Geometry check sheet. Reference: the model listing, model coordinates, mm. A direction names the side the tool comes from. Coordinates: 2 decimals unless noted, no trailing zeros. Write each loop counter-clockwise with the first axis right and the second up, starting at its lowest first coordinate (ties: lowest second). Pieces come first, ordered by that corner, then holes. Notation, with made-up numbers: M 44,59.5 L 83,59.5 A8 cw 83,63.5 Z; hole C 71,-5 d10. An arc over 180 degrees is marked long. Write each question's results on one line, items separated by ' | '.
```python
from build123d import *

# Parameters (mm, degrees)
SKETCH1_W           = 66
SKETCH1_H           = 54
BOSS_EXTRUDE1_DEPTH = 5
SKETCH2_R           = 2.5
SKETCH2_R_2         = 0.75
BOSS_EXTRUDE2_DEPTH = 4
SKETCH2_2_R         = 0.75
CUT_EXTRUDE1_DEPTH  = 4
CUT_EXTRUDE2_DEPTH  = 14
SKETCH4_R           = 1.6
SKETCH4_R_2         = 0.75
CUT_EXTRUDE3_DEPTH  = 5
CHAMFER1_SIZE       = 2
CUT_EXTRUDE4_START  = -66
SKETCH5_R           = 1.6
CUT_EXTRUDE4_DEPTH  = 10
SKETCH6_W           = 9.6
SKETCH6_H           = 16.5
CUT_EXTRUDE5_DEPTH  = 2.54


with BuildPart() as part:
    # Sketch1 → Boss-Extrude1 (new body)
    with BuildSketch(Plane.XY):
        Rectangle(SKETCH1_W, SKETCH1_H)
    extrude(amount=BOSS_EXTRUDE1_DEPTH)

    # Sketch2 → Boss-Extrude2 (add)
    with BuildSketch(Plane.XY.offset(5)):
        with Locations((28, -23)):
            Circle(SKETCH2_R)
        with Locations((28, -23)):
            Circle(SKETCH2_R_2, mode=Mode.SUBTRACT)
        with Locations((-28, -23)):
            Circle(SKETCH2_R)
        with Locations((-28, -23)):
            Circle(SKETCH2_R_2, mode=Mode.SUBTRACT)
        with Locations((-28, 23)):
            Circle(SKETCH2_R)
        with Locations((-28, 23)):
            Circle(SKETCH2_R_2, mode=Mode.SUBTRACT)
        with Locations((28, 23)):
            Circle(SKETCH2_R)
        with Locations((28, 23)):
            Circle(SKETCH2_R_2, mode=Mode.SUBTRACT)
        with BuildLine():
            Line((-25.5, 4), (-25.5, -4))
            ThreePointArc((-25.5, -4), (-28, -6.5), (-30.5, -4))
            Line((-30.5, -4), (-30.5, 4))
            ThreePointArc((-30.5, 4), (-28, 6.5), (-25.5, 4))
        make_face()
        with Locations((-28, -4)):
            Circle(SKETCH2_R_2, mode=Mode.SUBTRACT)
        with Locations((-28, 4)):
            Circle(SKETCH2_R_2, mode=Mode.SUBTRACT)
        with BuildLine():
            Line((25.5, 4), (25.5, -4))
            ThreePointArc((25.5, -4), (28, -6.5), (30.5, -4))
            Line((30.5, -4), (30.5, 4))
            ThreePointArc((30.5, 4), (28, 6.5), (25.5, 4))
        make_face()
        with Locations((28, -4)):
            Circle(SKETCH2_R_2, mode=Mode.SUBTRACT)
        with Locations((28, 4)):
            Circle(SKETCH2_R_2, mode=Mode.SUBTRACT)
    extrude(amount=BOSS_EXTRUDE2_DEPTH)

    # Sketch2<2> → Cut-Extrude1 (cut)
    with BuildSketch(Plane.XY.offset(5)):
        with Locations((-28, 23)):
            Circle(SKETCH2_2_R)
        with Locations((28, 23)):
            Circle(SKETCH2_2_R)
        with Locations((28, 4)):
            Circle(SKETCH2_2_R)
        with Locations((28, -4)):
            Circle(SKETCH2_2_R)
        with Locations((28, -23)):
            Circle(SKETCH2_2_R)
        with Locations((-28, -23)):
            Circle(SKETCH2_2_R)
        with Locations((-28, 4)):
            Circle(SKETCH2_2_R)
        with Locations((-28, -4)):
            Circle(SKETCH2_2_R)
    extrude(amount=-CUT_EXTRUDE1_DEPTH, mode=Mode.SUBTRACT)

    # Sketch3 → Cut-Extrude2 (cut)
    with BuildSketch(Plane.XY.offset(5)):
        with BuildLine():
            Line((-16.040925592, 12.723978191), (-5.394585654, 1.367882258))
            ThreePointArc((-5.394585654, 1.367882258), (-4.853660062, 0), (-5.394585654, -1.367882258))
            Line((-5.394585654, -1.367882258), (-16.040925592, -12.723978191))
            ThreePointArc((-16.040925592, -12.723978191), (-18.235476439, -13.21595464), (-19.5, -11.356095934))
            Line((-19.5, -11.356095934), (-19.5, 11.356095934))
            ThreePointArc((-19.5, 11.356095934), (-18.235476439, 13.21595464), (-16.040925592, 12.723978191))
        make_face()
        with BuildLine():
            Line((-10.958839938, 21), (10.958839938, 21))
            ThreePointArc((10.958839938, 21), (12.794019018, 19.795058326), (12.417914346, 17.632117742))
            Line((12.417914346, 17.632117742), (1.459074408, 5.942688475))
            ThreePointArc((1.459074408, 5.942688475), (0, 5.310570733), (-1.459074408, 5.942688475))
            Line((-1.459074408, 5.942688475), (-12.417914346, 17.632117742))
            ThreePointArc((-12.417914346, 17.632117742), (-12.794019018, 19.795058326), (-10.958839938, 21))
        make_face()
        with BuildLine():
            Line((5.394585654, -1.367882258), (16.040925592, -12.723978191))
            ThreePointArc((16.040925592, -12.723978191), (18.235476439, -13.21595464), (19.5, -11.356095934))
            Line((19.5, -11.356095934), (19.5, 11.356095934))
            ThreePointArc((19.5, 11.356095934), (18.235476439, 13.21595464), (16.040925592, 12.723978191))
            Line((16.040925592, 12.723978191), (5.394585654, 1.367882258))
            ThreePointArc((5.394585654, 1.367882258), (4.853660062, 0), (5.394585654, -1.367882258))
        make_face()
        with BuildLine():
            Line((12.417914346, -17.632117742), (1.459074408, -5.942688475))
            ThreePointArc((1.459074408, -5.942688475), (0, -5.310570733), (-1.459074408, -5.942688475))
            Line((-1.459074408, -5.942688475), (-12.417914346, -17.632117742))
            ThreePointArc((-12.417914346, -17.632117742), (-12.794019018, -19.795058326), (-10.958839938, -21))
            Line((-10.958839938, -21), (10.958839938, -21))
            ThreePointArc((10.958839938, -21), (12.794019018, -19.795058326), (12.417914346, -17.632117742))
        make_face()
    extrude(amount=-CUT_EXTRUDE2_DEPTH, mode=Mode.SUBTRACT)

    # Sketch4 → Cut-Extrude3 (cut)
    with BuildSketch(Plane.XZ.offset(27)):
        with Locations((-13, 2.5)):
            Circle(SKETCH4_R)
        with Locations((18, 2.5)):
            Circle(SKETCH4_R_2)
    extrude(amount=-CUT_EXTRUDE3_DEPTH, mode=Mode.SUBTRACT)

    # Chamfer1
    chamfer1_edges = [part.edges().sort_by_distance(p)[0] for p in [
        (6.938494377, -11.787403109, 0),
        (0, -5.310570733, 0),
        (-6.938494377, -11.787403109, 0),
        (-12.794019018, -19.795058326, 0),
        (0, -21, 0),
        (12.794019018, -19.795058326, 0),
        (-10.717755623, -7.045930225, 0),
        (-4.853660062, 0, 0),
        (-10.717755623, 7.045930225, 0),
        (-18.235476439, 13.21595464, 0),
        (-19.5, 0, 0),
        (-18.235476439, -13.21595464, 0),
        (10.717755623, -7.045930225, 0),
        (18.235476439, -13.21595464, 0),
        (19.5, 0, 0),
        (18.235476439, 13.21595464, 0),
        (10.717755623, 7.045930225, 0),
        (4.853660062, 0, 0),
        (6.938494377, 11.787403109, 0),
        (12.794019018, 19.795058326, 0),
        (0, 21, 0),
        (-12.794019018, 19.795058326, 0),
        (-6.938494377, 11.787403109, 0),
        (0, 5.310570733, 0),
        (0, 5.310570733, 5),
        (6.938494377, 11.787403109, 5),
        (12.794019018, 19.795058326, 5),
        (0, 21, 5),
        (-12.794019018, 19.795058326, 5),
        (-6.938494377, 11.787403109, 5),
        (4.853660062, 0, 5),
        (10.717755623, -7.045930225, 5),
        (18.235476439, -13.21595464, 5),
        (19.5, 0, 5),
        (18.235476439, 13.21595464, 5),
        (10.717755623, 7.045930225, 5),
        (-18.235476439, -13.21595464, 5),
        (-10.717755623, -7.045930225, 5),
        (-4.853660062, 0, 5),
        (-10.717755623, 7.045930225, 5),
        (-18.235476439, 13.21595464, 5),
        (-19.5, 0, 5),
        (12.794019018, -19.795058326, 5),
        (6.938494377, -11.787403109, 5),
        (0, -5.310570733, 5),
        (-6.938494377, -11.787403109, 5),
        (-12.794019018, -19.795058326, 5),
        (0, -21, 5),
    ]]
    chamfer(chamfer1_edges, length=CHAMFER1_SIZE)

    # Sketch5 → Cut-Extrude4 (cut)
    with BuildSketch(Plane.ZY.offset(33).offset(CUT_EXTRUDE4_START)):
        with Locations((2.5, 12)):
            Circle(SKETCH5_R)
    extrude(amount=CUT_EXTRUDE4_DEPTH, mode=Mode.SUBTRACT)

    # Sketch6 → Cut-Extrude5 (cut)
    with BuildSketch(Plane(origin=(0, 0, 0), x_dir=(-1, 0, 0), z_dir=(0, 0, -1))):
        with Locations((-28.2, -18.75)):
            Rectangle(SKETCH6_W, SKETCH6_H)
    extrude(amount=-CUT_EXTRUDE5_DEPTH, mode=Mode.SUBTRACT)


solid = part.part
```
Q1. Scan lines: probe 1 along Y at (x, z) = (28, 4.25); probe 2 along X at (y, z) = (20.5, 1.5); probe 3 along X at (y, z) = (-5, 4.75). Record each from-to range of solid material in increasing order.
Geometry check:
probe 1: y = -27 to -23.75, -22.25 to -4.75, -3.25 to 3.25, 4.75 to 22.25, 23.75 to 27 | probe 2: x = -33 to -12.96, 12.96 to 33 | probe 3: x = -33 to -21.25, -6.4 to -2.97, 2.97 to 6.4, 21.25 to 33
Q2. Sectioned sample at A-A on z = 6.25. Give the number of separate pieces and of enclosed holes in the cut face, and give its area (3 significant figures).
Geometry check:
separate pieces: 6 | enclosed holes: 8 | area: 184 mm2
Q3. Mould release check, pull along X, two halves, no side actions. Record for faces 1 (the flat face through (-30.5, 0, 7)), 2 (the conical face through (-18.47, -13.94, 3.76)): pulls with the +X half, pulls with the -X half, needs draft (parallel to the pull), parting line crosses it, or undercut.
Geometry check:
face 1: pulls with the -X half | face 2: undercut
Q4. Sectioned sample at D-D on x = -7. Record the cut outline in (y, z), and give its area (3 significant figures).
Geometry check:
outline: M -27,0 L -23,0 L -21,2 L -21,3 L -23,5 L -27,5 Z; M -11.85,2 L -8.93,0 L -6,0 L -3.08,2 L -3.08,3 L -6,5 L -8.93,5 L -11.85,3 Z; M 3.08,2 L 6,0 L 8.93,0 L 11.85,2 L 11.85,3 L 8.93,5 L 6,5 L 3.08,3 Z; M 21,2 L 23,0 L 27,0 L 27,5 L 23,5 L 21,3 Z | area: 116 mm2
Q5. Access from +Z, -Z, +X, -X, +Y, -Y to the whole of each face (thin tool, end or side, straight path). Record for faces 3 (the cylindrical face through (-12.807, -19.765, 2.507)), 4 (the flat face through (-7.581, -11.031, 1.014)), 5 (the cylindrical face through (-28.33, -20.52, 6.97)), 6 (the cylindrical face through (17.405, -24.535, 2.044)).
Geometry check:
face 3: +Z, -Z | face 4: -Z | face 5: +Z | face 6: -Y
Q6. Depth check by flat-ended pin: P1, Ø7.5, axis at x = 30, y = -22, coming from the -Z side; P2, Ø5, axis at x = -14.5, y = 8, coming from the +Z side; P3, Ø4, axis at x = -26, y = -14, coming from the +Z side; P4, Ø1.2, axis at x = 28, y = -23, coming from the +Z side. Enter the tip coordinate at first touch or a pass-through.
Geometry check:
P1: stops at z = 2.54 | P2: stops at z = 3.39 | P3: stops at z = 5 | P4: passes through
